CAD build for the part. Positions are in the model's coordinates, mm. A direction names the side the tool comes from. Coordinates: 2 decimals unless noted, no trailing zeros. Write each loop counter-clockwise with the first axis right and the second up, starting at its lowest first coordinate (ties: lowest second). Pieces come first, ordered by that corner, then holes. Notation, with made-up numbers: (24.5, -36.75) -> (73.5, -36.75) arc R18 cw to (73.5, -11.75) -> close; hole circle Ø6 at (1.25, 89). An arc over 180 degrees is marked (long way). Answer as CSV lines item,"result". Start each with the question number.
Autodesk Inventor part; units mm, degrees
ref_plane "YZ Plane" through (0, 0, 0) normal (1, 0, 0) x (0, 1, 0)
ref_plane "XZ Plane" through (0, 0, 0) normal (0, 1, 0) x (-1, 0, 0)
ref_plane "XY Plane" through (0, 0, 0) normal (0, 0, 1) x (1, 0, 0)
sketch "Sketch1" plane through (0, 0, 0) normal (0, 0, 1) x (1, 0, 0)
  line L0 (0, 0) -> (22.5, 0)
  line L1 (22.5, 0) -> (22.5, 23)
  line L2 (22.5, 23) -> (0, 23)
  line L3 (0, 23) -> (0, 0)
  dimension "d0" = 22.5
  dimension "d1" = 23
extrude "Extrusion1" add sketch "Sketch1" along normal blind 12.2
sketch "Sketch2" plane through (0, 0, 0) normal (0, -1, 0) x (1, 0, 0)
  line L0 (0, 12.2) -> (22.5, 12.2)
  line L1 (0, 0) -> (22.5, 0)
  line L2 (1.6, 12.2) -> (4.1, 12.2)
  line L3 (4.1, 12.2) -> (4.1, 0)
  line L4 (4.1, 0) -> (1.6, 0)
  line L5 (1.6, 0) -> (1.6, 12.2)
  line L6 (22.5, 0) -> (22.5, 12.2)
  dimension "d4" = 2.5
  dimension "d5" = 18.4
extrude "Extrusion2" add sketch "Sketch2" along normal blind 5 contours L0 L3 L1 L5
ref_plane "Work Plane1" through (22.5, 11.5, 0) normal (0, -1, 0) x (1, 0, 0)
mirror "Mirror1" about plane through (22.5, 11.5, 0) normal (0, -1, 0) of "Extrusion2"
ref_plane "Work Plane3" through (0, -2.5, 0) normal (0, -1, 0) x (1, 0, 0)
ref_plane "Work Plane4" through (0, 0, 6.1) normal (0, 0, 1) x (1, 0, 0)
hole "Hole1" at (1.6, -2.5, 6.1) direction (1, 0, 0) diameter 2 end through all
mirror "Mirror2" about plane through (22.5, 11.5, 0) normal (0, -1, 0) of "Hole1"
sketch "Sketch3" plane through (22.5, 0, 0) normal (0, -1, 0) x (1, 0, 0)
  line L0 (-4.7, 4.35) -> (-6, 4.35)
  line L1 (-6, 4.35) -> (-6, 7.85)
  line L2 (-6, 7.85) -> (-4.7, 7.85)
  line L3 (-4.7, 7.85) -> (-4.7, 4.35)
  line L4 (0, 12.2) -> (0, 0)
  line L5 (0, 0) -> (-18.4, 0)
  line L6 (-18.4, 12.2) -> (-18.4, 0)
  line L7 (-20.9, 12.2) -> (-18.4, 12.2)
  line L8 (-20.9, 0) -> (-20.9, 12.2)
  line L9 (-20.9, 0) -> (-22.5, 0)
  line L10 (-22.5, 0) -> (-22.5, 12.2)
  line L11 (-22.5, 12.2) -> (-20.9, 12.2)
  line L12 (-18.4, 12.2) -> (0, 12.2)
  line L13 (-18.4, 0) -> (-20.9, 0)
  line L14 (0, 12.2) -> (0, 0)
  line L15 (0, 0) -> (-18.4, 0)
  line L16 (-18.4, 12.2) -> (-18.4, 0)
  line L17 (-20.9, 12.2) -> (-18.4, 12.2)
  line L18 (-20.9, 0) -> (-20.9, 12.2)
  line L19 (-20.9, 0) -> (-22.5, 0)
  line L20 (-22.5, 0) -> (-22.5, 12.2)
  line L21 (-22.5, 12.2) -> (-20.9, 12.2)
  line L22 (-18.4, 12.2) -> (0, 12.2)
  line L23 (-18.4, 0) -> (-20.9, 0)
  line L24 (0, 12.2) -> (0, 0)
  line L25 (0, 0) -> (-18.4, 0)
  line L26 (-18.4, 12.2) -> (-18.4, 0)
  line L27 (-20.9, 12.2) -> (-18.4, 12.2)
  line L28 (-20.9, 0) -> (-20.9, 12.2)
  line L29 (-20.9, 0) -> (-22.5, 0)
  line L30 (-22.5, 0) -> (-22.5, 12.2)
  line L31 (-22.5, 12.2) -> (-20.9, 12.2)
  line L32 (-18.4, 12.2) -> (0, 12.2)
  line L33 (-18.4, 0) -> (-20.9, 0)
  line L34 (-27, 6.1) -> (4.5, 6.1)
  point P0 (-6, 6.1)
  dimension "d17" = 1.3
  dimension "d18" = 3.5
  dimension "d19" = 4.7
extrude "Extrusion3" add sketch "Sketch3" along normal blind 2 contours L0 L1 L34 L3 | L34 L1 L2 L3
sketch "Sketch4" plane through (0, 0, 0) normal (-1, 0, 0) x (0, 0, 1)
  line L0 (6.1, 34.6) -> (6.1, -11.6)
  circle A0 centre (6.1, 6.1) radius 6.1
  line L1 (0, 0) -> (0, 23)
  line L2 (0, 0) -> (12.2, 0)
extrude "Extrusion4" add sketch "Sketch4" along normal blind 5.8 contours A0 L0 | L0 A0
sketch "Sketch5" plane through (-5.8, 6.1, 6.1) normal (-1, 0, 0) x (0, 0, 1)
  circle A0 centre (0, 0) radius 2
  point P0 (-6.1, -6.1)
  dimension "d24" = 4
extrude "Extrusion5" add sketch "Sketch5" along normal blind 3.25
sketch "Sketch6" plane through (0, 23, 0) normal (-1, 0, 0) x (0, 0, 1)
  circle A0 centre (6.1, -16.9) radius 6.1
  arc A1 (12.2, -16.9) -> (0, -16.9) centre (6.1, -16.9) ccw
  circle A2 centre (6.1854, -10.8006) radius 2.5717
  point P0 (0, -23)
extrude "Extrusion6" add sketch "Sketch6" along normal up to surface (5.8 mm away) contours A2 A0 | A0 A2 picked at (5.289, -10.1215) picked at (6.9125, -11.6556)
ref_plane "Work Plane2" through (22.5, 11.5, 0) normal (0, -1, 0) x (1, 0, 0)
properties part number "servo_metal_600TVL"
1. Flat gauge pins, fed straight in: P1, Ø1.5, axis at x = -5.5, z = 4, coming from the +Y side; P2, Ø5.5, axis at y = 24.5, z = 7, coming from the -X side; P3, Ø0.7, axis at x = 17, y = -1, coming from the +Z side; P4, Ø1.5, axis at x = -1.5, y = 21, coming from the +Z side. Where does each tip first touch, or does it go through?
2. Cut at B-B (z = 5.5). Count the separate pieces of the cut face and the enclosed holes in it, then the cut area to 3 significant figures.
3. Tool access for faces 1 (the face through (1, 23, 6)), 2 (the face through (-7.402, 5.499, 8.008)), 3 (the face through (4.1, -1, 6)): list every direction of +Z, -Z, +X, -X, +Y, -Y with a clear straight run to the whole face (end or side of a thin tool).
4. Cut at C-C (x = 17). Give the cut face in (y, z), then the cut area to 3 significant figures.
5. Cut at A-A (y = 25.5). Give the cut face in (x, z), then the cut area to 3 significant figures.
6. Cut at D-D (z = 2.5). Give the cut face in (x, y), then the cut area to 3 significant figures.
7. Wall check: line 1 (Y direction, x = 2.6, z = 6.1); line 2 (Z direction, x = 2.55, y = 25.5); line 3 (X direction, y = 20.5, z = 9.75). Give the ranges that are in metal, low to high.
8. Mould opens along Z. For faces 4 (the face through (22.5, 11, 6)), 5 (the face through (11, 12, 0)), 6 (the face through (2.867, -2.8, 7.054)) say: pulls with the +Z half, pulls with the -Z half, needs draft (parallel to the pull), parting line crosses it, or undercut.
Geometry check:
1,P1,"y = 14.33"
1,P2,"x = 0"
1,P3,"z = 7.85"
1,P4,"through"
2,separate pieces,"3"
2,enclosed holes,"0"
2,area,"634 mm²"
3,face 1,"+Z, -Z, -X, +Y"
3,face 2,"-X"
3,face 3,"+Z, -Z, -Y"
4,outline,"(-2, 4.35) -> (0, 4.35) -> (0, 0) -> (23, 0) -> (23, 12.2) -> (0, 12.2) -> (0, 7.85) -> (-2, 7.85) -> close"
4,area,"288 mm²"
5,outline,"(1.6, 0) -> (4.1, 0) -> (4.1, 5.1) -> (1.6, 5.1) -> close; (1.6, 7.1) -> (4.1, 7.1) -> (4.1, 12.2) -> (1.6, 12.2) -> close"
5,area,"25.5 mm²"
6,outline,"(-5.8, 1.18) -> (0, 1.18) -> (0, 0) -> (1.6, 0) -> (1.6, -5) -> (4.1, -5) -> (4.1, 0) -> (22.5, 0) -> (22.5, 23) -> (4.1, 23) -> (4.1, 28) -> (1.6, 28) -> (1.6, 23) -> (0, 23) -> (0, 11.02) -> (-5.8, 11.02) -> close"
6,area,"600 mm²"
7,line 1,"-5 to -3.5, -1.5 to 24.5, 26.5 to 28"
7,line 2,"0 to 5.1, 7.1 to 12.2"
7,line 3,"0 to 22.5"
8,face 4,"needs draft"
8,face 5,"pulls with the -Z half"
8,face 6,"undercut"
